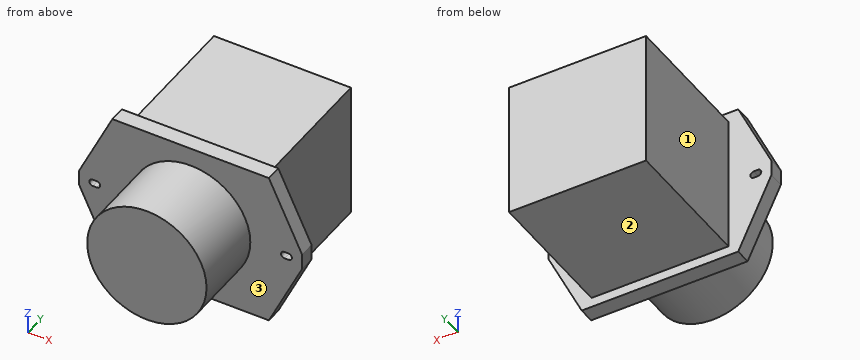
Autodesk Fusion 360 part; units mm, degrees
sketch "Sketch1" plane through (0, 0, 0) normal (0, 1, 0) x (1, 0, 0)
  line L0 (-73.5, -97.2411) -> (-23.5, -97.2411)
  line L1 (-72.5, -97.2411) -> (-24.5, -97.2411) construction
  line L2 (-77, -97.2411) -> (-20, -97.2411) construction
  line L3 (-48.5, -117.2411) -> (-48.5, -77.2411)
  line L4 (-23.5, -96.3461) -> (-24.5, -96.3461)
  arc A0 (-24.5, -96.3461) -> (-24.5, -98.1361) centre (-24.5, -97.2411) ccw
  line L5 (-24.5, -98.1361) -> (-23.5, -98.1361)
  arc A1 (-23.5, -98.1361) -> (-23.5, -96.3461) centre (-23.5, -97.2411) ccw
  line L6 (-23.5, -97.2411) -> (-24.5, -97.2411) construction
  line L7 (-72.5, -96.3461) -> (-73.5, -96.3461)
  arc A2 (-73.5, -96.3461) -> (-73.5, -98.1361) centre (-73.5, -97.2411) ccw
  line L8 (-73.5, -98.1361) -> (-72.5, -98.1361)
  arc A3 (-72.5, -98.1361) -> (-72.5, -96.3461) centre (-72.5, -97.2411) ccw
  line L9 (-72.5, -97.2411) -> (-73.5, -97.2411) construction
  circle A4 centre (-48.5, -97.2411) radius 15.2574
  line L10 (-31, -114.7411) -> (-66, -114.7411)
  line L11 (-66, -114.7411) -> (-66, -79.7411)
  line L12 (-66, -79.7411) -> (-31, -79.7411)
  line L13 (-31, -79.7411) -> (-31, -114.7411)
  line L14 (-48.5, -114.7411) -> (-48.5, -79.7411) construction
  line L15 (-31, -97.2411) -> (-66, -97.2411) construction
  line L16 (-68.5, -117.2411) -> (-28.5, -117.2411)
  line L17 (-28.5, -117.2411) -> (-28.5, -77.2411) construction
  line L18 (-28.5, -77.2411) -> (-68.5, -77.2411)
  line L19 (-68.5, -77.2411) -> (-68.5, -117.2411) construction
  line L20 (-68.5, -97.2411) -> (-28.5, -97.2411) construction
  line L21 (-68.5, -117.2411) -> (-77, -99.2411)
  line L22 (-77, -99.2411) -> (-77, -97.2411)
  line L23 (-77, -97.2411) -> (-77, -95.2411)
  line L24 (-77, -95.2411) -> (-68.5, -77.2411)
  line L25 (-28.5, -117.2411) -> (-20, -99.2411)
  line L26 (-20, -99.2411) -> (-20, -97.2411)
  line L27 (-20, -97.2411) -> (-20, -95.2411)
  line L28 (-20, -95.2411) -> (-28.5, -77.2411)
  dimension "d1" = 50
  dimension "d2" = 48
  dimension "d3" = 57
  dimension "d4" = 40
  dimension "d5" = 1.79
  dimension "d6" = 1.79
  dimension "d7" = 35
  dimension "d8" = 35
  dimension "d9" = 40
  dimension "d10" = 40
  dimension "d11" = 4
extrude "Extrude1" add sketch "Sketch1" along normal blind 35 contours L0 L3 A4 L11 L12 | L0 L3 A4 L10 L11 | L0 L3 A4 | L0 L3 A4 | L0 L3 A4 | L0 L3 A4 | L0 L3 A4 L12 L13 | L0 L3 A4 L10 L13
extrude "Extrude2" add sketch "Sketch1" against normal blind 4
extrude "Extrude3" add sketch "Sketch1" against normal blind 22.6 contours L0 L3 A4 | L0 L3 A4 | L0 L3 A4 | L0 L3 A4
equation "d16 = -26.6 mm + 4 mm"
The model under review builds one solid part; all positions refer to its coordinate system, in mm. Face numbers are marked on the shaded views. A direction names the side the tool comes from. Give positions to 0.01 mm unless a question says otherwise; leave off trailing zeros. Loops run counter-clockwise (first coordinate to the right, second up) from the corner with the lowest first, then second, coordinate; pieces in that order, holes last. Notation, with made-up numbers: (7.25, 23) -> (15.25, 23) arc R28 ccw to (15.25, 51) -> close; hole circle Ø6 at (-13.5, 2). An arc over 180 degrees is marked (long way). Use CSV: the item, a comma, the result in double quotes.
1. Consider section C-C, the plane y = 10. Write out the cut boundary in (x, z).
Result:
outline,"(-66, 79.74) -> (-31, 79.74) -> (-31, 114.74) -> (-66, 114.74) -> close"
2. For P1, Ø0.8, axis at x = -73, y = -2, coming from the -Z side; P2, Ø5, axis at y = 7, z = 84.5, coming from the +X side; P3, Ø8, axis at y = 15.5, z = 109.5, coming from the -X side; P4, Ø4, axis at x = -39.5, y = 1, coming from the +Z side, all flat-tipped, find the tip position at first contact; note any pin that passes through.
Result:
P1,"stops at z = 85.92"
P2,"stops at x = -31"
P3,"stops at x = -66"
P4,"stops at z = 117.24"
3. Machinability: for the marked faces 1, 2 and 3, which of the approach directions +Z, -Z, +X, -X, +Y, -Y give a long, thin tool a straight path to every point of the face, cutting with its end or side? Answer none if there is none.
Result:
face 1,"+Z, -Z, -X, +Y"
face 2,"-Z, +X, -X, +Y"
face 3,"-Y"
4. To check wall thickness, follow probe 1 along Z at (x, y) = (-39.5, 31.5); probe 2 along X at (y, z) = (17.5, 102); probe 3 along Y at (x, z) = (-69, 104). State the ranges of each line that lie inside material, in increasing order. Write a range as from..to.
Result:
probe 1,"z = 79.74..114.74"
probe 2,"x = -66..-31"
probe 3,"y = -4..0"
5. Consider section B-B, the plane z = 87. Write out the cut boundary in (x, y), then the cut area to 3 significant figures.
Result:
outline,"(-73.11, -4) -> (-59.81, -4) -> (-59.81, -22.6) -> (-37.19, -22.6) -> (-37.19, -4) -> (-23.89, -4) -> (-23.89, 0) -> (-31, 0) -> (-31, 35) -> (-66, 35) -> (-66, 0) -> (-73.11, 0) -> close"
area,"1,840 mm²"
6. Consider section D-D, the plane x = -65. Write out the cut boundary in (y, z), then the cut area to 4 significant figures.
Result:
outline,"(-4, 77.24) -> (0, 77.24) -> (0, 79.74) -> (35, 79.74) -> (35, 114.74) -> (0, 114.74) -> (0, 117.24) -> (-4, 117.24) -> close"
area,"1,385 mm²"
7. Consider section A-A, the plane x = -48.5. Write out the cut boundary in (y, z), then the cut area to 3 significant figures.
Result:
outline,"(-22.6, 81.98) -> (-4, 81.98) -> (-4, 77.24) -> (0, 77.24) -> (0, 79.74) -> (35, 79.74) -> (35, 114.74) -> (0, 114.74) -> (0, 117.24) -> (-4, 117.24) -> (-4, 112.5) -> (-22.6, 112.5) -> close"
area,"1,950 mm²"
